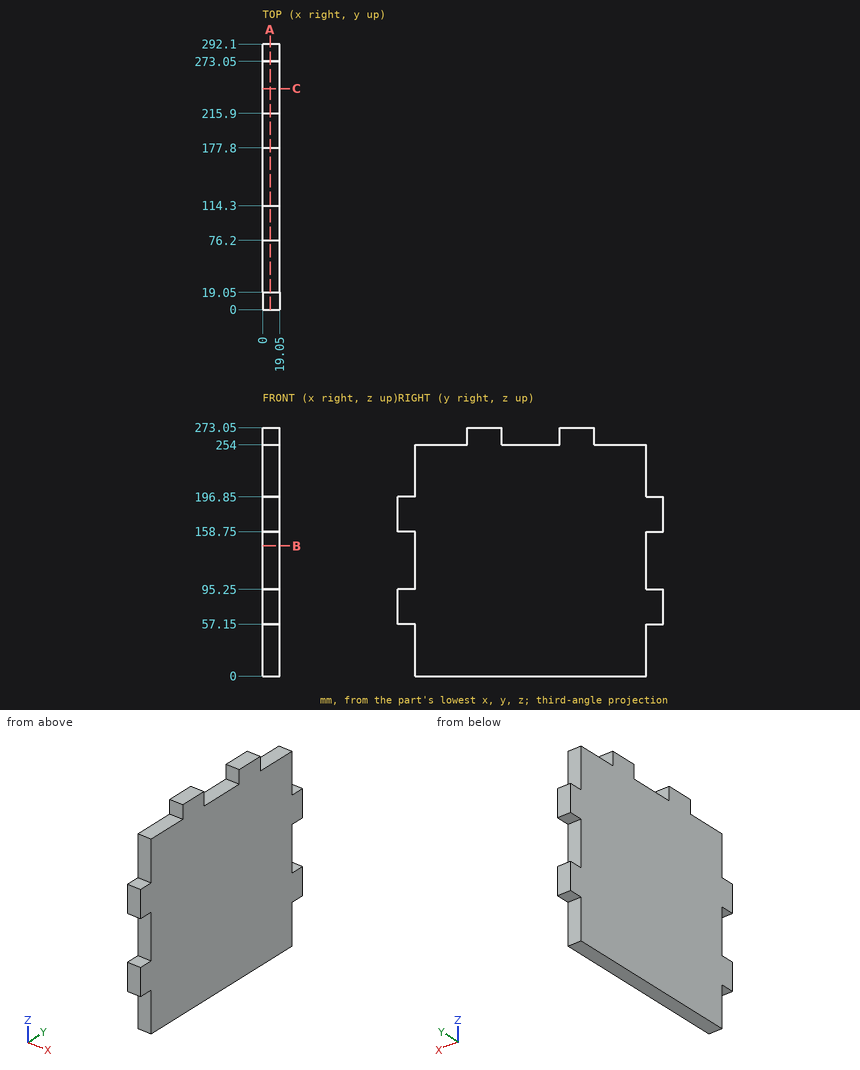
Check sheet for the drawn part. Datum: minimum x, y, z corner. Units: mm. Round coordinates to 2 decimals unless told otherwise and drop trailing zeros. Loops run counter-clockwise (first coordinate to the right, second up) from the corner with the lowest first, then second, coordinate; pieces in that order, holes last.
Item 1: Cross-section at A-A on x = 8.5. Record the boundary of the cut face in (y, z).
Item 2: Cross-section at C-C on y = 243. Record the boundary of the cut face in (x, z).
Item 3: Cross-section at B-B on z = 143. Record the boundary of the cut face in (x, y).
Item 4: Thickness scan on line 1 (Z direction, x = 13.75, y = 14); line 2 (Z direction, x = 3.25, y = 56); line 3 (Y direction, x = 18, z = 135). Record the ranges inside material, lowest first.
Item 5: Gauge pin test, flat ends, axial feed: pin 1 (9.5 mm diameter, centred on x = 13, y = 281, fed in from -Z); pin 2 (1 mm diameter, centred on x = 8.5, y = 79.5, fed in from -Z); pin 3 (10 mm diameter, centred on x = 12.5, z = 148, fed in from +Y); pin 4 (5 mm diameter, centred on x = 6, y = 147.5, fed in from +Z). Record the tip position at first contact, or that the pin passes through.
Answer sheet:
1. outline: (0, 57.15) - (19.05, 57.15) - (19.05, 0) - (273.05, 0) - (273.05, 57.15) - (292.1, 57.15) - (292.1, 95.25) - (273.05, 95.25) - (273.05, 158.75) - (292.1, 158.75) - (292.1, 196.85) - (273.05, 196.85) - (273.05, 254) - (215.9, 254) - (215.9, 273.05) - (177.8, 273.05) - (177.8, 254) - (114.3, 254) - (114.3, 273.05) - (76.2, 273.05) - (76.2, 254) - (19.05, 254) - (19.05, 196.85) - (0, 196.85) - (0, 158.75) - (19.05, 158.75) - (19.05, 95.25) - (0, 95.25) - close
2. outline: (0, 0) - (19.05, 0) - (19.05, 254) - (0, 254) - close
3. outline: (0, 19.05) - (19.05, 19.05) - (19.05, 273.05) - (0, 273.05) - close
4. line 1: z = 57.15 to 95.25, 158.75 to 196.85
4. line 2: z = 0 to 254
4. line 3: y = 19.05 to 273.05
5. pin 1: stops at z = 57.15
5. pin 2: stops at z = 0
5. pin 3: stops at y = 273.05
5. pin 4: stops at z = 254
